from build123d import *

# Parameters (mm, degrees)
F1_W     = 25
F1_H     = 5
F1_R     = 1.25
F2_DEPTH = 2
F0_W     = 15
F0_H     = 3
F3_DEPTH = 1
F5_DEPTH = 2
F6_R     = 2


with BuildPart() as f2:
    # F1 (on Front) → F2 (new body)
    with BuildSketch(Plane.XZ):
        with Locations((0.7514315657, 15.9062612424)):
            Rectangle(F1_W, F1_H)
        with Locations((-9.2485684343, 15.9062612424)):
            Circle(F1_R, mode=Mode.SUBTRACT)
        with Locations((10.7514315657, 15.9062612424)):
            Circle(F1_R, mode=Mode.SUBTRACT)
    extrude(amount=F2_DEPTH)

    # F0 (on Front) → F3 (cut)
    with BuildSketch(Plane.XZ):
        with Locations((0.7514315657, 16.9062612424)):
            Rectangle(F0_W, F0_H)
    extrude(amount=F3_DEPTH, mode=Mode.SUBTRACT)

    # F4 (on Front) → F5 (join)
    with BuildSketch(Plane.XZ):
        with BuildLine():
            ThreePointArc((11.7901169805, 15.2108242509), (10.058409027, 14.8659633231), (9.7095267544, 16.5968655894))
            Line((9.7095267544, 16.5968655894), (0.7694446684, 3.1090927712))
            Line((0.7694446684, 3.1090927712), (2.2445774484, 0.8925128366))
            Line((2.2445774484, 0.8925128366), (11.7901169805, 15.2108242509))
        make_face()
        Polygon((2.2445774484, 0.8925128366), (0.7694446684, 3.1090927712), (-0.7182862862, 0.8645745513), (0.7534939653, -1.3441127186), align=None)
        with BuildLine():
            Line((-0.7182862862, 0.8645745513), (0.7694446684, 3.1090927712))
            Line((0.7694446684, 3.1090927712), (-8.207945318, 16.5987953787))
            ThreePointArc((-8.207945318, 16.5987953787), (-8.4991860984, 14.9057982922), (-10.2057692667, 15.1023541792))
            Line((-10.2057692667, 15.1023541792), (-0.7182862862, 0.8645745513))
        make_face()
        with BuildLine():
            Line((10.5591020697, -11.6011478636), (2.2445774484, 0.8925128366))
            Line((2.2445774484, 0.8925128366), (0.7534939653, -1.3441127186))
            Line((0.7534939653, -1.3441127186), (8.5106430868, -12.9851960237))
            ThreePointArc((8.5106430868, -12.9851960237), (9.3518197991, -12.0222448757), (10.5591020697, -11.6011478636))
        make_face()
        with BuildLine():
            Line((0.7534939653, -1.3441127186), (-0.7182862862, 0.8645745513))
            Line((-0.7182862862, 0.8645745513), (-8.9852317039, -11.6076466904))
            ThreePointArc((-8.9852317039, -11.6076466904), (-7.8193399291, -12.0425669267), (-7.0075444884, -12.9856721197))
            Line((-7.0075444884, -12.9856721197), (0.7534939653, -1.3441127186))
        make_face()
        with BuildLine():
            Line((11.6190981521, -13.1939306142), (10.5591020697, -11.6011478636))
            ThreePointArc((10.5591020697, -11.6011478636), (9.3518197991, -12.0222448757), (8.5106430868, -12.9851960237))
            Line((8.5106430868, -12.9851960237), (9.7112213616, -14.7868929477))
            ThreePointArc((9.7112213616, -14.7868929477), (9.9502917065, -13.1342206879), (11.6190981521, -13.1939306142))
        make_face()
        with BuildLine():
            ThreePointArc((13.2514315657, -14.0937387576), (12.4498390934, -12.259232865), (10.5591020697, -11.6011478636))
            Line((10.5591020697, -11.6011478636), (11.6190981521, -13.1939306142))
            ThreePointArc((11.6190981521, -13.1939306142), (11.9018843533, -13.6049050604), (12.0014315657, -14.0937387576))
            ThreePointArc((12.0014315657, -14.0937387576), (11.1135346207, -15.2901422754), (9.7112213616, -14.7868929477))
            Line((9.7112213616, -14.7868929477), (8.5106430868, -12.9851960237))
            ThreePointArc((8.5106430868, -12.9851960237), (10.1822089367, -16.5280734919), (13.2514315657, -14.0937387576))
        make_face()
        with BuildLine():
            Line((-9.9451010739, -13.0557877559), (-8.9852317039, -11.6076466904))
            ThreePointArc((-8.9852317039, -11.6076466904), (-11.1071084292, -15.7658120476), (-6.7485684343, -14.0937387576))
            ThreePointArc((-6.7485684343, -14.0937387576), (-6.8141732461, -13.5247747274), (-7.0075444884, -12.9856721197))
            Line((-7.0075444884, -12.9856721197), (-8.208505519, -14.7871139319))
            ThreePointArc((-8.208505519, -14.7871139319), (-10.1311078637, -14.9789642404), (-9.9451010739, -13.0557877559))
        make_face()
        with BuildLine():
            ThreePointArc((-7.0075444884, -12.9856721197), (-7.8193399291, -12.0425669267), (-8.9852317039, -11.6076466904))
            Line((-8.9852317039, -11.6076466904), (-9.9451010739, -13.0557877559))
            ThreePointArc((-9.9451010739, -13.0557877559), (-8.6604212586, -12.9907505891), (-7.9985684343, -14.0937387576))
            ThreePointArc((-7.9985684343, -14.0937387576), (-8.0522033888, -14.4559689026), (-8.208505519, -14.7871139319))
            Line((-8.208505519, -14.7871139319), (-7.0075444884, -12.9856721197))
        make_face()
    extrude(amount=F5_DEPTH)

    # F6
    f6_edges = [f2.edges().sort_by_distance(p)[0] for p in [
        (0.769445, -1, 3.109093),
        (-0.718286, -1, 0.864575),
        (2.244577, -1, 0.892513),
        (0.753494, -1, -1.344113),
        (7.594703, -1, 13.406261),
        (-6.083316, -1, 13.406261),
        (-9.075561, -1, 13.406261),
        (10.587075, -1, 13.406261),
    ]]
    fillet(f6_edges, radius=F6_R)


solid = f2.part
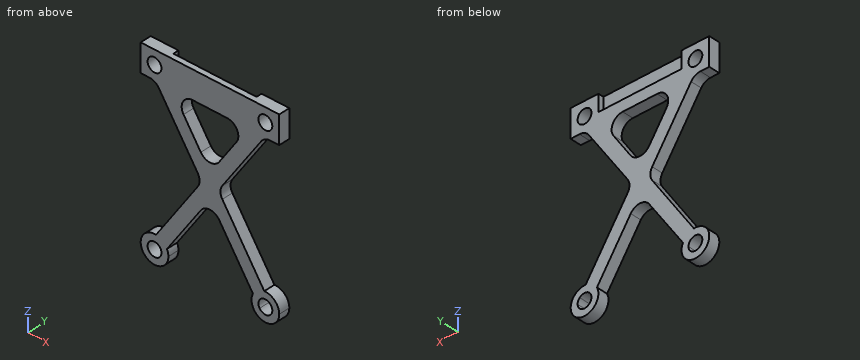
Part model, mm, in its own coordinate system. Give positions to 0.01 mm unless a question says otherwise; leave off trailing zeros. Order: outer loops, then holes, each group sorted by start corner. A loop starts at its lowest first (then second) coordinate and runs counter-clockwise, first axis right, second up. Notation, with made-up numbers: (48.25, -19) -> (71.25, -19) arc R17 cw to (71.25, 8) -> close; hole circle Ø10 at (2.5, -22). An arc over 180 degrees is marked (long way). Use one line per item in the form item = value.
(1) Saw through at C-C (x = -2). Write the cut outline in (y, z).
Solution:
outline = (-2, -5.47) -> (0, -5.47) -> (0, -1.07) -> (-2, -1.07) -> close; (-2, 2.79) -> (0, 2.79) -> (0, 7.27) -> (-2, 7.27) -> close; (-2, 13.41) -> (0, 13.41) -> (0, 15.41) -> (-1, 15.41) -> (-1, 18.41) -> (-2, 18.41) -> close
(2) Saw through at B-B (z = -9.5). Write the cut outline in (x, y), then the cut area to 3 significant figures.
Solution:
outline = (-7.59, -2) -> (-4.68, -2) -> (-4.68, 0) -> (-7.59, 0) -> close; (6.19, -2) -> (9.16, -2) -> (9.16, 0) -> (6.19, 0) -> close
area = 11.8 mm²
(3) Saw through at A-A (x = -6). Write the cut outline in (y, z), then the cut area to 3 significant figures.
Solution:
outline = (-2, -11.47) -> (0, -11.47) -> (0, -7.1) -> (-2, -7.1) -> close; (-2, 8.79) -> (0, 8.79) -> (0, 15.41) -> (-1, 15.41) -> (-1, 18.41) -> (-2, 18.41) -> close
area = 25.0 mm²
(4) Drill centre lines: line 1 (X direction, y = -0.2, z = 17); line 2 (Z direction, x = 10, y = -1.2); line 3 (Z direction, x = 5, y = -0.6). Where is each one in solid material? Low to high. Write a range as from..to.
Solution:
line_1 = -11.75..-9.85, -8.64..-6.75, 8.25..10.15, 11.36..13.25
line_2 = -16.48..-15.09, -13.09..-10.76, 12.53..14.91, 16.91..18.41
line_3 = -7.72..-3.25, 5.03..9.49, 13.06..15.41
(5) Saw through at D-D (x = 11). Write the cut outline in (y, z), then the cut area to 3 significant figures.
Solution:
outline = (-2, -16.58) -> (0, -16.58) -> (0, -15.32) -> (-2, -15.32) -> close; (-2, -12.87) -> (0, -12.87) -> (0, -11.61) -> (-2, -11.61) -> close; (-2, 13.3) -> (0, 13.3) -> (0, 14.68) -> (-2, 14.68) -> close; (-2, 17.13) -> (0, 17.13) -> (0, 18.41) -> (-2, 18.41) -> close
area = 10.4 mm²
